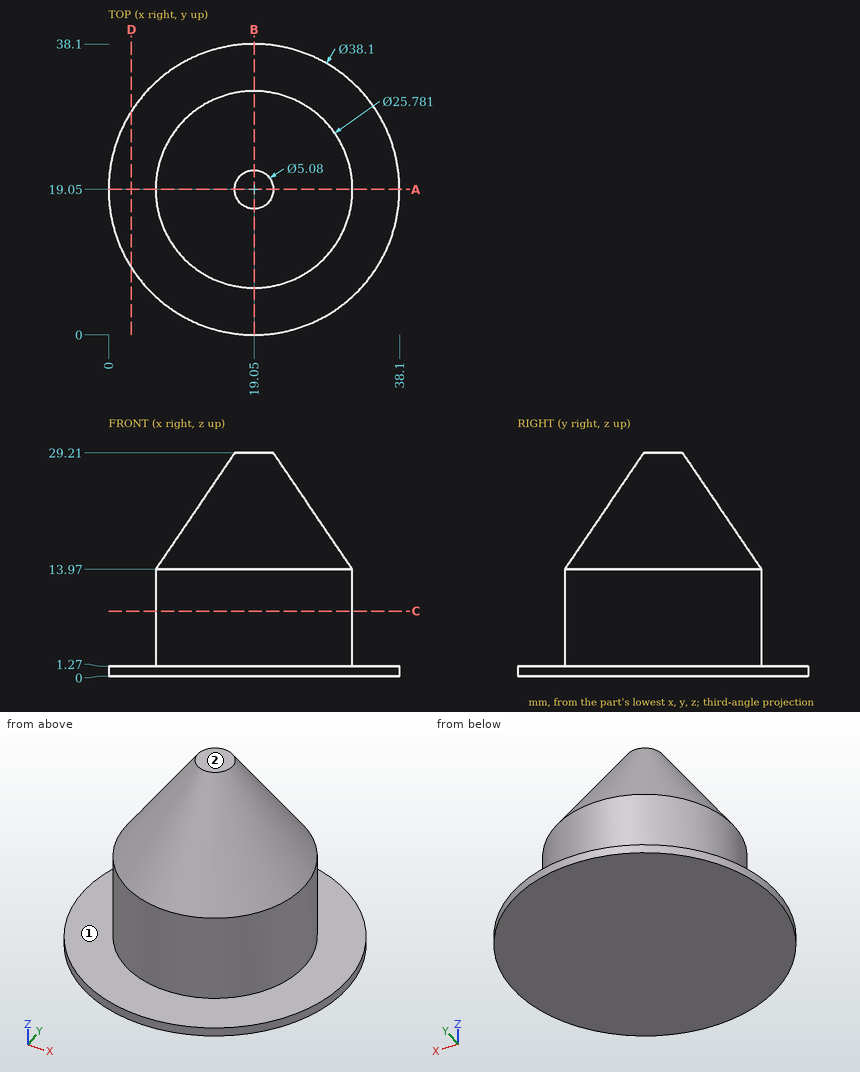
Can you work these out from the drawing? Everything is in mm from the part's minimum corner. A direction names the side the tool comes from. Give positions to 0.01 mm unless a question says otherwise; leave off trailing zeros. Loops run counter-clockwise (first coordinate to the right, second up) from the corner with the lowest first, then second, coordinate; pieces in that order, holes last. Notation, with made-up numbers: (55.5, 10.5) -> (75.5, 10.5) arc R21 ccw to (75.5, 19.5) -> close; hole circle Ø1 at (73, 65.5). An arc over 180 degrees is marked (long way). Return JSON: item names as keys, results as strings.
Q1. I want a section at C-C, the plane z = 8.5. List the corners of the cut face in (x, y) for me.
Checks:
{"outline": "circle Ø25.78 at (19.05, 19.05)"}
Q2. I need wall thicknesses on probe 1 along Z at (x, y) = (29.5, 4); probe 2 along Z at (x, y) = (28.5, 26.5); probe 3 along Y at (x, z) = (19, 18.5). Which ranges of each line are inside material? Lowest first, please.
Checks:
{"probe 1": "z = 0 to 1.27", "probe 2": "z = 0 to 15.23", "probe 3": "y = 9.24 to 28.86"}
Q3. I want a section at D-D, the plane x = 3. List the corners of the cut face in (y, z) for me.
Checks:
{"outline": "(8.79, 0) -> (29.31, 0) -> (29.31, 1.27) -> (8.79, 1.27) -> close"}
Q4. For pin 1 Ø2 at (x, y) = (23.5, 13) entering from +Z; pin 2 Ø5 at (x, y) = (32, 32) entering from -Z; pin 3 Ø5 at (y, z) = (7.5, 22) entering from +X; pin 4 Ø12 at (x, z) = (15.5, 12.5) entering from -Y, each with a flat end and sliding along its axis, tell me the tip position at first contact or that it passes through.
Checks:
{"pin 1": "stops at z = 23.36", "pin 2": "stops at z = 0", "pin 3": "passes through", "pin 4": "stops at y = 6.16"}
Q5. I want a section at A-A, the plane y = 19.05. List the corners of the cut face in (x, z) for me.
Checks:
{"outline": "(0, 0) -> (38.1, 0) -> (38.1, 1.27) -> (31.94, 1.27) -> (31.94, 13.97) -> (21.59, 29.21) -> (16.51, 29.21) -> (6.16, 13.97) -> (6.16, 1.27) -> (0, 1.27) -> close"}
Q6. On a 3-axis mill with a long thin cutter (end or side, diameter ignored), from which of +Z, -Z, +X, -X, +Y, -Y can I reach the whole of each face in a straight line? I mean the marked faces 1 and 2. Say none if no direction works.
Checks:
{"face 1": "+Z", "face 2": "+Z, +X, -X, +Y, -Y"}
